For this review, take the finished solid that the model builds, in its own axes (mm). A direction names the side the tool comes from. Round coordinates to 2 decimals unless told otherwise and drop trailing zeros. Order: outer loops, then holes, each group sorted by start corner. A loop starts at its lowest first (then second) coordinate and runs counter-clockwise, first axis right, second up. Notation, with made-up numbers: M 27,22.25 L 40,22.25 A32 ccw 40,56.25 Z; hole C -39,40 d10. An arc over 180 degrees is marked long. Use a Markdown table: item, result.
from build123d import *

# Parameters (mm, degrees)
EXTRUDE_THIN1_DEPTH        = 45
CHAMFER1_SIZE              = 15
CONVERT_SOLID1_DEPTH       = 45
CONVERT_SOLID1_2_DEPTH     = 45
FILLET1_R                  = 2
FILLET2_R                  = 10
F_6_5_6_5_DIAMETER_HOLE1_D = 6.5
F_6_5_6_5_DIAMETER_HOLE2_D = 6.5


# Read off the part's stored shape, not the designer's step: Convert-Solid1
with BuildPart() as part:
    # Sketch1 → Extrude-Thin1 (new body)
    with BuildSketch(Plane(origin=(0, 0, 0), x_dir=(1, 0, 0), z_dir=(0, 1, 0))):
        Polygon((-159, 75), (-159, 0), (159, 0), (159, 75), (155, 75), (155, 4), (-155, 4), (-155, 75), align=None)
    extrude(amount=EXTRUDE_THIN1_DEPTH)

    # Chamfer1
    chamfer1_edges = [part.edges().sort_by_distance(p)[0] for p in [
        (-157, 45, -75),
        (157, 45, -75),
    ]]
    chamfer(chamfer1_edges, length=CHAMFER1_SIZE)

    # Convert-Solid1 outline → Convert-Solid1 (cut)
    with BuildSketch(Plane(origin=(0, 0, 0), x_dir=(1, 0, 0), z_dir=(0, 1, 0))):
        with BuildLine():
            Line((-159, 0), (-153, 0))
            ThreePointArc((-153, 0), (-157.242640687, 1.757359313), (-159, 6))
            Line((-159, 6), (-159, 0))
        make_face()
        with BuildLine():
            ThreePointArc((159, 6), (157.242640687, 1.757359313), (153, 0))
            Line((153, 0), (159, 0))
            Line((159, 0), (159, 6))
        make_face()
    extrude(amount=CONVERT_SOLID1_DEPTH, mode=Mode.SUBTRACT)

    # Convert-Solid1 2 outline → Convert-Solid1 2 (add)
    with BuildSketch(Plane(origin=(0, 0, 0), x_dir=(1, 0, 0), z_dir=(0, 1, 0))):
        with BuildLine():
            Line((-155, 4), (-153, 4))
            ThreePointArc((-153, 4), (-154.414213562, 4.585786438), (-155, 6))
            Line((-155, 6), (-155, 4))
        make_face()
        with BuildLine():
            ThreePointArc((155, 6), (154.414213562, 4.585786438), (153, 4))
            Line((153, 4), (155, 4))
            Line((155, 4), (155, 6))
        make_face()
    extrude(amount=CONVERT_SOLID1_2_DEPTH)

    # Fillet1
    fillet1_edges = [part.edges().sort_by_distance(p)[0] for p in [
        (157, 0, -75),
        (-157, 0, -75),
    ]]
    fillet(fillet1_edges, radius=FILLET1_R)

    # Fillet2
    fillet2_edges = [part.edges().sort_by_distance(p)[0] for p in [
        (157, 30, -75),
        (157, 45, -60),
        (-157, 45, -60),
        (-157, 30, -75),
    ]]
    fillet(fillet2_edges, radius=FILLET2_R)

    # Ø6.5 (6.5) Diameter Hole1 (through all)
    with Locations(Plane(origin=(-159, 22, -202.5), x_dir=(0, 0, 1), z_dir=(-1, 0, 0))):
        with Locations((-178.5, -12), (-142.5, -12), (142.5, -12), (178.5, -12)):
            Hole(F_6_5_6_5_DIAMETER_HOLE1_D / 2)

    # Ø6.5 (6.5) Diameter Hole2 (through all)
    with Locations(Plane(origin=(159, 22, -202.5), x_dir=(0, 0, -1), z_dir=(1, 0, 0))):
        with Locations((-178.5, -12), (-142.5, -12), (142.5, -12), (178.5, -12)):
            Hole(F_6_5_6_5_DIAMETER_HOLE2_D / 2)


solid = part.part
Q1. Machinability: for faces 4 (the flat face through (2, 22, -4)), 5 (the flat face through (159, 22, -40)), which of the approach directions +Z, -Z, +X, -X, +Y, -Y give a long, thin tool a straight path to every point of the face, cutting with its end or side? Answer none if there is none.
Determined:
| item | result |
|---|---|
| face 4 | -Z, +Y, -Y |
| face 5 | +Z, -Z, +X, +Y, -Y |
Q2. Draft analysis for pull direction Y (two halves, no side actions). For faces 1 (the flat face through (-1, 0, -2)), 2 (the flat face through (-157, 38, -67)), 3 (the cylindrical face through (-156.972, 10.143, -56.753)), state which applies: pulls with the +Y half, pulls with the -Y half, needs draft (parallel to the pull), parting line crosses it, or undercut.
Determined:
| item | result |
|---|---|
| face 1 | pulls with the -Y half |
| face 2 | pulls with the +Y half |
| face 3 | undercut |
Q3. Add section D-D (x = 6.5). Write out the cut boundary in (y, z), then the cut area to 3 significant figures.
Determined:
| item | result |
|---|---|
| outline | M 0,-4 L 45,-4 L 45,0 L 0,0 Z |
| area | 180 mm^2 |
Q4. Add section B-B (z = -68). Write out the cut boundary in (x, y).
Determined:
| item | result |
|---|---|
| outline | M -159,0 L -155,0 L -155,37 L -159,37 Z; M 155,0 L 159,0 L 159,37 L 155,37 Z |
Q5. Clearance check with a flat-ended pin moving along its axis: pin 1 (8 mm diameter, centred on x = 18, y = 29, fed in from -Z). State where the tip first meets the part, or that it passes through.
Determined:
| item | result |
|---|---|
| pin 1 | stops at z = -4 |
Q6. Wall thickness on line 1 along X through (y, z) = (34, -65); line 2 along Y through (x, z) = (-156.95, -24); line 3 along Z through (x, y) = (-155.85, 10): over which ranges is each line inside the solid? List them lowest first. Write a range as [from, to].
Determined:
| item | result |
|---|---|
| line 1 | x = [-159, -155], [155, 159] |
| line 2 | y = [0, 6.75], [13.25, 45] |
| line 3 | z = [-75, -63.25], [-56.75, -27.25], [-20.75, -0.72] |
Q7. Add section C-C (y = 10). Write out the cut boundary in (x, z).
Determined:
| item | result |
|---|---|
| outline | M -159,-75 L -155,-75 L -155,-63.25 L -159,-63.25 Z; M -159,-56.75 L -155,-56.75 L -155,-27.25 L -159,-27.25 Z; M -159,-20.75 L -155,-20.75 L -155,-6 A2 cw -153,-4 L 153,-4 A2 cw 155,-6 L 155,-20.75 L 159,-20.75 L 159,-6 A6 ccw 153,0 L -153,0 A6 ccw -159,-6 Z; M 155,-75 L 159,-75 L 159,-63.25 L 155,-63.25 Z; M 155,-56.75 L 159,-56.75 L 159,-27.25 L 155,-27.25 Z |
Q8. Add section A-A (z = -24). Write out the cut boundary in (x, y), then the cut area to 3 significant figures.
Determined:
| item | result |
|---|---|
| outline | M -159,0 L -155,0 L -155,6.75 L -159,6.75 Z; M -159,13.25 L -155,13.25 L -155,45 L -159,45 Z; M 155,0 L 159,0 L 159,6.75 L 155,6.75 Z; M 155,13.25 L 159,13.25 L 159,45 L 155,45 Z |
| area | 308 mm^2 |
